```python
from build123d import *

# Parameters (mm, degrees)
CROQUIS1_W              = 30
CROQUIS1_H              = 75
CROQUIS1_R              = 2.05
CROQUIS1_R_2            = 2.55
SALIENTE_EXTRUIR1_DEPTH = 5
CROQUIS4_R              = 4.05
CORTAR_EXTRUIR1_DEPTH   = 2.8
CROQUIS5_W              = 30
CROQUIS5_H              = 17.7
SALIENTE_EXTRUIR2_DEPTH = 5
REDONDEO1_R             = 4


with BuildPart() as part:
    # Croquis1 → Saliente-Extruir1 (new body)
    with BuildSketch(Plane.XY):
        with Locations((15, 37.5)):
            Rectangle(CROQUIS1_W, CROQUIS1_H)
        with Locations((5, 66.8)):
            Circle(CROQUIS1_R, mode=Mode.SUBTRACT)
        with Locations((25, 66.8)):
            Circle(CROQUIS1_R, mode=Mode.SUBTRACT)
        with Locations((25, 46.8)):
            Circle(CROQUIS1_R, mode=Mode.SUBTRACT)
        with Locations((5, 46.8)):
            Circle(CROQUIS1_R, mode=Mode.SUBTRACT)
        with Locations((15, 11.08)):
            Circle(CROQUIS1_R_2, mode=Mode.SUBTRACT)
    extrude(amount=SALIENTE_EXTRUIR1_DEPTH)

    # Croquis4 → Cortar-Extruir1 (cut)
    with BuildSketch(Plane.XY.offset(5)):
        with Locations((5, 66.8)):
            Circle(CROQUIS4_R)
        with Locations((5, 46.8)):
            Circle(CROQUIS4_R)
        with Locations((25, 46.8)):
            Circle(CROQUIS4_R)
        with Locations((25, 66.8)):
            Circle(CROQUIS4_R)
    extrude(amount=-CORTAR_EXTRUIR1_DEPTH, mode=Mode.SUBTRACT)

    # Croquis5 → Saliente-Extruir2 (add, through all)
    with BuildSketch(Plane.XY.offset(5)):
        with Locations((15, -8.85)):
            Rectangle(CROQUIS5_W, CROQUIS5_H)
    extrude(amount=-SALIENTE_EXTRUIR2_DEPTH)

    # Redondeo1
    redondeo1_edges = [part.edges().sort_by_distance(p)[0] for p in [
        (0, -17.7, 2.5),
        (30, -17.7, 2.5),
        (0, 75, 2.5),
        (30, 75, 2.5),
    ]]
    fillet(redondeo1_edges, radius=REDONDEO1_R)


solid = part.part
```
Verification items for the finished model (mm, model axes). A direction names the side the tool comes from. Round coordinates to 2 decimals unless told otherwise and drop trailing zeros. Write each loop counter-clockwise with the first axis right and the second up, starting at its lowest first coordinate (ties: lowest second). Pieces come first, ordered by that corner, then holes. Notation, with made-up numbers: (72.25, 63.25) -> (91.25, 63.25) arc R9 ccw to (91.25, 75.25) -> close; hole circle Ø2 at (8.25, -3.5). An arc over 180 degrees is marked (long way). Write each question's results on one line, items separated by ' | '.
Q1. Draft check along Y on faces 3 (the face through (15, -17.7, 3)), 4 (the face through (4.556, 44.799, 1.085)), 5 (the face through (28.859, 73.797, 2.535)). Enter one of: released by +Y, released by -Y, zero draft, split by the parting line, or undercut.
Derived:
face 3: released by -Y | face 4: undercut | face 5: released by +Y
Q2. Sectioned sample at C-C, the plane y = 66.8. Record the boundary of the cut face in (x, z), and give its area (3 significant figures).
Derived:
outline: (0, 0) -> (2.95, 0) -> (2.95, 2.2) -> (0.95, 2.2) -> (0.95, 5) -> (0, 5) -> close; (7.05, 0) -> (22.95, 0) -> (22.95, 2.2) -> (20.95, 2.2) -> (20.95, 5) -> (9.05, 5) -> (9.05, 2.2) -> (7.05, 2.2) -> close; (27.05, 0) -> (30, 0) -> (30, 5) -> (29.05, 5) -> (29.05, 2.2) -> (27.05, 2.2) -> close | area: 86.6 mm²
Q3. Sectioned sample at B-B, the plane x = 15. Record the boundary of the cut face in (y, z), and give its area (3 significant figures).
Derived:
outline: (-17.7, 0) -> (8.53, 0) -> (8.53, 5) -> (-17.7, 5) -> close; (13.63, 0) -> (75, 0) -> (75, 5) -> (13.63, 5) -> close | area: 438 mm²
Q4. Thickness scan on probe 1 along X at (y, z) = (66.8, 1.6); probe 2 along Y at (x, z) = (25, 4.2); probe 3 along Y at (x, z) = (25, 0.85). Record the ranges inside material, lowest first.
Derived:
probe 1: x = 0 to 2.95, 7.05 to 22.95, 27.05 to 30 | probe 2: y = -17.7 to 42.75, 50.85 to 62.75, 70.85 to 75 | probe 3: y = -17.7 to 44.75, 48.85 to 64.75, 68.85 to 75
Q5. Sectioned sample at D-D, the plane z = 3.95. Record the boundary of the cut face in (x, y).
Derived:
outline: (0, -13.7) arc R4 ccw to (4, -17.7) -> (26, -17.7) arc R4 ccw to (30, -13.7) -> (30, 71) arc R4 ccw to (26, 75) -> (4, 75) arc R4 ccw to (0, 71) -> close; hole circle Ø8.1 at (5, 46.8); hole circle Ø8.1 at (5, 66.8); hole circle Ø5.1 at (15, 11.08); hole circle Ø8.1 at (25, 46.8); hole circle Ø8.1 at (25, 66.8)
Q6. Sectioned sample at A-A, the plane x = 5. Record the boundary of the cut face in (y, z).
Derived:
outline: (-17.7, 0) -> (44.75, 0) -> (44.75, 2.2) -> (42.75, 2.2) -> (42.75, 5) -> (-17.7, 5) -> close; (48.85, 0) -> (64.75, 0) -> (64.75, 2.2) -> (62.75, 2.2) -> (62.75, 5) -> (50.85, 5) -> (50.85, 2.2) -> (48.85, 2.2) -> close; (68.85, 0) -> (75, 0) -> (75, 5) -> (70.85, 5) -> (70.85, 2.2) -> (68.85, 2.2) -> close
Q7. Access from +Z, -Z, +X, -X, +Y, -Y to the whole of each face (thin tool, end or side, straight path). Record for faces 1 (the face through (4.122, 62.846, 3.62)), 2 (the face through (15, 29, 5)).
Derived:
face 1: +Z | face 2: +Z, +X, -X, +Y, -Y
Q8. Go/stop test with a flat-tipped pin: pin 1 Ø2.5 at (x, y) = (24, 46.5) entering from +Z. Record where the tip stops, or that it passes through.
Derived:
pin 1: stops at z = 2.2
